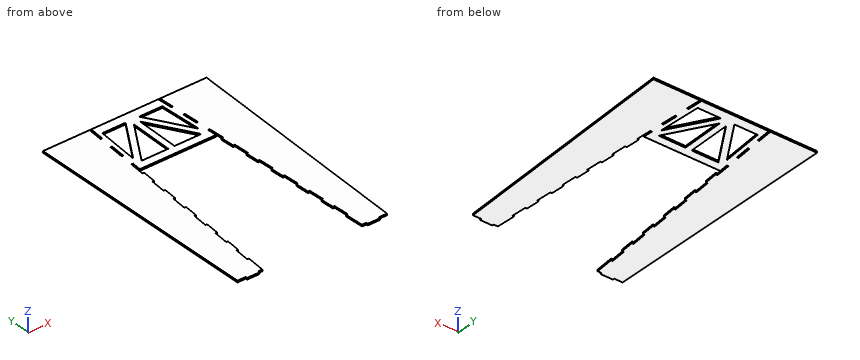
```python
from build123d import *

# Parameters (mm, degrees)
BOSS_EXTRUDE1_DEPTH = 10.16
CUT_EXTRUDE5_DEPTH  = 12.7


with BuildPart() as part:
    # Sketch1 → Boss-Extrude1 (new body)
    with BuildSketch(Plane.XY):
        Polygon((-502.783260205, 1465.163333881), (-459.721789204, 17.476365817), (-408.921789204, 17.476365817), (-408.921789204, 7.316365817), (-332.100796745, 7.316365817), (-332.100796745, 17.476365817), (-306.627827519, 17.476365817), (-234.627172097, 1054.1), (234.627172097, 1054.1), (306.627827519, 17.476365817), (332.721789205, 17.476365817), (332.721789205, 7.316365817), (408.921789205, 7.316365817), (408.921789205, 17.476365817), (459.721789204, 17.476365817), (502.783260205, 1465.163333881), align=None)
        Polygon((183.241684323, 1104.9), (19.05, 1104.9), (19.05, 1370.513438368), align=None, mode=Mode.SUBTRACT)
        Polygon((-184.672467887, 1406.743333881), (-41.445883295, 1406.743333881), (-202.80261453, 1145.716008632), align=None, mode=Mode.SUBTRACT)
        Polygon((-19.05, 1370.513438368), (-19.05, 1104.9), (-183.241684323, 1104.9), align=None, mode=Mode.SUBTRACT)
        Polygon((184.672467887, 1406.743333881), (202.80261453, 1145.716008632), (41.445883295, 1406.743333881), align=None, mode=Mode.SUBTRACT)
    extrude(amount=BOSS_EXTRUDE1_DEPTH)

    # Sketch2 → Cut-Extrude5 (cut)
    with BuildSketch(Plane.XY):
        Polygon((-222.69422447, 1372.274878096), (-212.576544386, 1371.572135487), (-206.36877838, 1460.947946306), (-216.535268781, 1460.947946306), align=None)
        Polygon((-224.894455765, 1194.225999066), (-235.012135849, 1194.928741675), (-228.490407278, 1288.824803216), (-218.372727194, 1288.122060607), align=None)
        Polygon((224.894455765, 1194.225999066), (235.012135849, 1194.928741675), (228.490407278, 1288.824803216), (218.372727194, 1288.122060607), align=None)
        Polygon((212.576544386, 1371.572135487), (222.694224471, 1372.274878096), (216.535268781, 1460.947946306), (206.36877838, 1460.947946306), align=None)
        Polygon((-240.810161517, 1111.452134365), (-247.330047228, 1017.582605255), (-237.212367144, 1016.879862645), (-230.692481433, 1110.749391756), align=None)
        Polygon((237.212367144, 1016.879862645), (247.330047228, 1017.582605255), (240.810161517, 1111.452134365), (230.692481433, 1110.749391756), align=None)
        Polygon((-298.801924037, 130.149180543), (-292.291252627, 223.886047498), (-302.408932711, 224.588790108), (-308.919604121, 130.851923152), align=None)
        Polygon((-243.012235672, 933.376722904), (-253.129915756, 934.079465513), (-259.647958606, 840.236468834), (-249.530278522, 839.533726225), align=None)
        Polygon((243.012235672, 933.376722904), (253.129915756, 934.079465513), (259.647958606, 840.236468834), (249.530278522, 839.533726225), align=None)
        Polygon((-274.16610128, 484.841453384), (-284.283781364, 485.544195993), (-277.769424233, 579.334127811), (-267.651744149, 578.631385201), align=None)
        Polygon((-261.848189901, 662.187589804), (-271.965869985, 662.890332413), (-265.449669994, 756.706796662), (-255.33198991, 756.004054053), align=None)
        Polygon((261.848189901, 662.187589804), (271.965869985, 662.890332413), (265.449669994, 756.706796662), (255.33198991, 756.004054053), align=None)
        Polygon((274.16610128, 484.841453384), (284.283781364, 485.544195993), (277.769424233, 579.334127811), (267.651744149, 578.631385201), align=None)
        Polygon((-286.484012658, 307.495316963), (-296.601692742, 308.198059572), (-290.089178472, 401.961458959), (-279.971498388, 401.25871635), align=None)
        Polygon((286.484012658, 307.495316963), (296.601692742, 308.198059572), (290.089178472, 401.961458959), (279.971498388, 401.25871635), align=None)
        Polygon((298.801924037, 130.149180543), (308.919604121, 130.851923152), (302.408932711, 224.588790108), (292.291252627, 223.886047498), align=None)
    extrude(amount=CUT_EXTRUDE5_DEPTH, mode=Mode.SUBTRACT)


solid = part.part
```
Can you work these out from the model? Positions are in its coordinate system, mm. Round coordinates to 2 decimals unless told otherwise and drop trailing zeros. Loops run counter-clockwise (first coordinate to the right, second up) from the corner with the lowest first, then second, coordinate; pieces in that order, holes last. Notation, with made-up numbers: (32, 41.5) -> (77, 41.5) arc R18 cw to (77, 52.5) -> close; hole circle Ø1 at (40, 56.25). An arc over 180 degrees is marked (long way). Answer in a Markdown table with one row per item.
Item 1: If I drill on probe 1 along Y at (x, z) = (103, 9.5); probe 2 along Y at (x, z) = (112.5, 1.75); probe 3 along X at (y, z) = (1142, 9), over which ranges is the centre line in solid material (lowest first)?
Answer block:
| item | result |
|---|---|
| probe 1 | 1054.1 to 1104.9, 1234.71 to 1307.17, 1406.74 to 1465.16 |
| probe 2 | 1054.1 to 1104.9, 1219.34 to 1291.8, 1406.74 to 1465.16 |
| probe 3 | -493.17 to -160.31, -19.05 to 19.05, 160.31 to 493.17 |
Item 2: Will these pins go through, and if not, where does the flat tip stop? P1, Ø4, axis at y = 1086, z = 6, coming from the +X side; P2, Ø3, axis at y = 596.5, z = 6, coming from the +X side; P3, Ø3, axis at x = 446, z = 5.5, coming from the -Y side.
Answer block:
| item | result |
|---|---|
| P1 | x = 491.56 |
| P2 | x = 476.99 |
| P3 | y = 17.48 |
Item 3: Suppose I cut it at A-A, the plane y = 387. List the corners of the cut face in (x, z) for me, plus the area to 3 significant figures.
Answer block:
| item | result |
|---|---|
| outline | (-470.71, 0) -> (-291.13, 0) -> (-291.13, 10.16) -> (-470.71, 10.16) -> close; (291.13, 0) -> (470.71, 0) -> (470.71, 10.16) -> (291.13, 10.16) -> close |
| area | 3,650 mm² |
Item 4: Suppose I cut it at D-D, the plane z = 8. Give the number of separate pieces and of enclosed holes in the cut face, plus the area to 3 significant figures.
Answer block:
| item | result |
|---|---|
| separate pieces | 1 |
| enclosed holes | 8 |
| area | 738,000 mm² |
Item 5: Suppose I cut it at C-C, the plane y = 1222. List the corners of the cut face in (x, z) for me, plus the area to 3 significant figures.
Answer block:
| item | result |
|---|---|
| outline | (-495.55, 0) -> (-233.13, 0) -> (-233.13, 10.16) -> (-495.55, 10.16) -> close; (-222.97, 0) -> (-197.5, 0) -> (-197.5, 10.16) -> (-222.97, 10.16) -> close; (-155.65, 0) -> (-110.86, 0) -> (-110.86, 10.16) -> (-155.65, 10.16) -> close; (-19.05, 0) -> (19.05, 0) -> (19.05, 10.16) -> (-19.05, 10.16) -> close; (110.86, 0) -> (155.65, 0) -> (155.65, 10.16) -> (110.86, 10.16) -> close; (197.5, 0) -> (222.97, 0) -> (222.97, 10.16) -> (197.5, 10.16) -> close; (233.13, 0) -> (495.55, 0) -> (495.55, 10.16) -> (233.13, 10.16) -> close |
| area | 7,150 mm² |
Item 6: Suppose I cut it at B-B, the plane x = 153.5. List the corners of the cut face in (y, z) for me.
Answer block:
| item | result |
|---|---|
| outline | (1054.1, 0) -> (1104.9, 0) -> (1104.9, 10.16) -> (1054.1, 10.16) -> close; (1153.01, 0) -> (1225.47, 0) -> (1225.47, 10.16) -> (1153.01, 10.16) -> close; (1406.74, 0) -> (1465.16, 0) -> (1465.16, 10.16) -> (1406.74, 10.16) -> close |
